Verification items for this drawing (mm, ordinates from the low corner). A direction names the side the tool comes from. Round coordinates to 2 decimals unless told otherwise and drop trailing zeros. Order: outer loops, then holes, each group sorted by start corner. A loop starts at its lowest first (then second) coordinate and runs counter-clockwise, first axis right, second up. Notation, with made-up numbers: (71.25, 23) - (99.25, 23) arc R16 cw to (99.25, 44) - close; hole circle Ø9 at (-31, 67). An arc over 180 degrees is marked (long way). Use a Markdown table: item, result. Add a question column.
(1) Section check B-B on z = 37.5. Record the boundary of the cut face in (x, y), then the cut area to 3 significant figures.
(2) Mould release check, pull along X, two halves, no side actions. Record for the marked faces 1, 2 and 3: released by +X, released by -X, zero draft, split by the parting line, or undercut.
(3) Section check D-D on x = 38.5. Record the boundary of the cut face in (y, z), then the cut area to 3 significant figures.
(4) Section check A-A on y = 2.5. Record the boundary of the cut face in (x, z).
(5) Gauge pin test, flat ends, axial feed: P1, Ø2, axis at y = 4.5, z = 31, coming from the -X side (3 decimals); P2, Ø12.5, axis at x = 25, z = 25, coming from the +Y side; P3, Ø3, axis at x = 41, y = 4, coming from the -Z side (1 decimal); P4, Ø2, axis at x = 38.5, y = 6.5, coming from the -Z side. Record the tip position at first contact, or that the pin passes through.
(6) Section check C-C on y = 8.5. Record the boundary of the cut face in (x, z).
(7) Access from +Z, -Z, +X, -X, +Y, -Y to the whole of each face (thin tool, end or side, straight path). Record for the marked faces 4 and 5.
(8) Thickness scan on line 1 along Z through (x, y) = (25, 1.7); line 2 along X through (y, z) = (2.3, 5). Record the ranges inside material, lowest first. Write a range as [from, to].
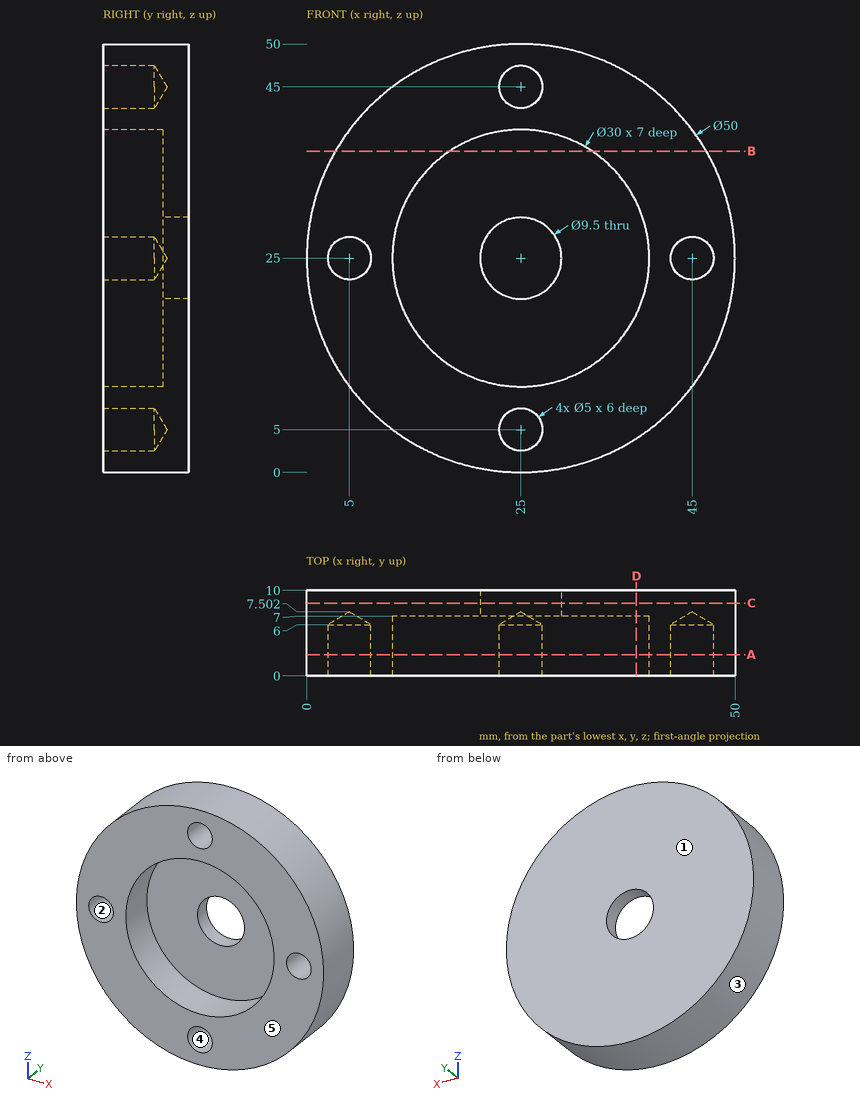
Check sheet entries:
| question | item | result |
|---|---|---|
| 1 | outline | (3.35, 0) - (16.71, 0) - (16.71, 7) - (33.29, 7) - (33.29, 0) - (46.65, 0) - (46.65, 10) - (3.35, 10) - close |
| 1 | area | 317 mm2 |
| 2 | face 1 | zero draft |
| 2 | face 2 | undercut |
| 2 | face 3 | split by the parting line |
| 3 | outline | (0, 3.96) - (10, 3.96) - (10, 46.04) - (0, 46.04) - (0, 31.54) - (7, 31.54) - (7, 18.46) - (0, 18.46) - close |
| 3 | area | 329 mm2 |
| 4 | outline | circle Ø50 at (25, 25); hole circle Ø5 at (5, 25); hole circle Ø30 at (25, 25); hole circle Ø5 at (25, 5); hole circle Ø5 at (25, 45); hole circle Ø5 at (45, 25) |
| 5 | P1 | stops at x = 0.505 |
| 5 | P2 | stops at y = 10 |
| 5 | P3 | stops at z = 4.6 |
| 5 | P4 | stops at z = 3.35 |
| 6 | outline | circle Ø50 at (25, 25); hole circle Ø9.5 at (25, 25) |
| 7 | face 4 | -Y |
| 7 | face 5 | +Z, -Z, +X, -X, -Y |
| 8 | line 1 | z = [0, 2.5], [7.5, 10], [40, 42.5], [47.5, 50] |
| 8 | line 2 | x = [10, 22.5], [27.5, 40] |
